```python
from build123d import *

# Parameters (mm, degrees)
F0_R     = 27.400357
F2_DEPTH = 1.778
F1_R     = 17.246114
F3_DEPTH = 1.778
F6_DEPTH = 1.778
F7_COUNT = 5


with BuildPart() as f2:
    # F0 (on Top) → F2 (new body)
    with BuildSketch(Plane.XY):
        Circle(F0_R)
    extrude(amount=F2_DEPTH)

    # F1 (on Top) → F3 (cut, through all)
    with BuildSketch(Plane.XY):
        Circle(F1_R)
    extrude(amount=F3_DEPTH, mode=Mode.SUBTRACT)


with BuildPart() as f6:
    # F5 (on Top) → F6 (new body, through all)
    with BuildSketch(Plane.XY):
        with BuildLine():
            Line((-0.888398, 20.0147), (-0.864621, 20.042582))
            ThreePointArc((-0.864621, 20.042582), (-0.87662, 20.028736), (-0.888398, 20.0147))
        make_face()
        with BuildLine():
            Line((3.656133, 25.34403), (-0.864621, 20.042582))
            Line((-0.864621, 20.042582), (-0.888398, 20.0147))
            ThreePointArc((-0.888398, 20.0147), (-0.765731, 18.420441), (0.831965, 18.484277))
            Line((0.831965, 18.484277), (0.917938, 18.585037))
            Line((0.917938, 18.585037), (5.409154, 23.848715))
            ThreePointArc((5.409154, 23.848715), (5.280411, 25.473012), (3.656133, 25.34403))
        make_face()
        with BuildLine():
            Line((0.917938, 18.585037), (0.831965, 18.484277))
            ThreePointArc((0.831965, 18.484277), (0.876401, 18.53342), (0.917938, 18.585037))
        make_face()
    extrude(amount=F6_DEPTH)


with BuildPart() as f7_1:
    # F7: instance of F6
    add(f6.part.rotate(Axis((0, 0, 1.187779), (0, 0, -1)), 1 * 360 / F7_COUNT))


with BuildPart() as f7_2:
    # F7: instance of F6
    add(f6.part.rotate(Axis((0, 0, 1.187779), (0, 0, -1)), 2 * 360 / F7_COUNT))


with BuildPart() as f7_3:
    # F7: instance of F6
    add(f6.part.rotate(Axis((0, 0, 1.187779), (0, 0, -1)), 3 * 360 / F7_COUNT))


with BuildPart() as f7_4:
    # F7: instance of F6
    add(f6.part.rotate(Axis((0, 0, 1.187779), (0, 0, -1)), 4 * 360 / F7_COUNT))


with BuildPart() as f2_1:
    add(f2.part)

    # F8: cut F6, F7_1, F7_2, F7_3, F7_4
    add(f6.part, mode=Mode.SUBTRACT)
    add(f7_1.part, mode=Mode.SUBTRACT)
    add(f7_2.part, mode=Mode.SUBTRACT)
    add(f7_3.part, mode=Mode.SUBTRACT)
    add(f7_4.part, mode=Mode.SUBTRACT)


solid = f2_1.part
```
Could you check a few things on this model? Use its own coordinates, in mm. Coordinates: 2 decimals unless noted, no trailing zeros. Write each loop counter-clockwise with the first axis right and the second up, starting at its lowest first coordinate (ties: lowest second). Pieces come first, ordered by that corner, then holes. Notation, with made-up numbers: (17, 85.5) -> (39, 85.5) arc R15 cw to (39, 109.5) -> close; hole circle Ø9 at (-25, 55.5). An arc over 180 degrees is marked (long way). Write item = value, one per line. Start each with the question number.
(1) I want a section at A-A (y = 0). Please give me the cut outline in (x, z).
(2) I want a section at D-D (x = 2). Please give me the cut outline in (y, z), plus the area to 3 significant figures.
(3) Will this pin go through, and if not, where does the flat tip stop? pin 1 (1 mm diameter, centred on x = -17, z = 0.5, fed in from +Y).
(4) I need wall thicknesses on line 1 (Y direction, x = 0, z = 0.5); line 2 (Y direction, x = 5.5, z = 0.9); line 3 (Y direction, x = 18, z = 0.8). Which ranges of each line are inside material? Lowest first, please. Write a range as [from, to].
(5) We'd pull the mould along Y, two halves only. Please class faces 1 (the face through (18, 0, 0)), 2 (the face through (-20.195, 18.518, 0.877)), 3 (the face through (25.85, 2.83, 0.88)): released by +Y, released by -Y, zero draft, split by the parting line, or undercut.
(6) I want a section at C-C (z = 0.7). Give the number of separate pieces and of enclosed holes in the cut face, plus the area to 3 significant figures.
(7) I want a section at B-B (x = 23). Please give me the cut outline in (y, z), plus the area to 3 significant figures.
Result set:
q1.outline = (-27.4, 0) -> (-17.25, 0) -> (-17.25, 1.78) -> (-27.4, 1.78) -> close; (17.25, 0) -> (27.4, 0) -> (27.4, 1.78) -> (17.25, 1.78) -> close
q2.outline = (-27.33, 0) -> (-17.13, 0) -> (-17.13, 1.78) -> (-27.33, 1.78) -> close; (17.13, 0) -> (19.85, 0) -> (19.85, 1.78) -> (17.13, 1.78) -> close; (23.4, 0) -> (27.33, 0) -> (27.33, 1.78) -> (23.4, 1.78) -> close
q2.area = 30.0 mm2
q3.pin_1 = 21.88
q4.line_1 = [-27.4, -17.25], [17.25, 18.13], [21.06, 27.4]
q4.line_2 = [-26.84, -16.35], [16.35, 23.97], [25.22, 26.84]
q4.line_3 = [-20.66, 4.85], [7.06, 20.66]
q5.face_1 = zero draft
q5.face_2 = split by the parting line
q5.face_3 = undercut
q6.separate_pieces = 1
q6.enclosed_holes = 6
q6.area = 1,320 mm2
q7.outline = (-14.89, 0) -> (2.78, 0) -> (2.78, 1.78) -> (-14.89, 1.78) -> close; (5.28, 0) -> (14.89, 0) -> (14.89, 1.78) -> (5.28, 1.78) -> close
q7.area = 48.5 mm2
